Autodesk Inventor part; units mm, degrees
ref_plane "Plano de trabajo1" through (0, 0, 0) normal (0, 0, 1) x (1, 0, 0)
ref_plane "YZ Plane" through (0, 0, 0) normal (1, 0, 0) x (0, 1, 0)
ref_plane "XZ Plane" through (0, 0, 0) normal (0, 1, 0) x (-1, 0, 0)
ref_plane "Plano de trabajo1" through (0, 0, 0) normal (0, 0, 1) x (1, 0, 0)
sketch "Boceto1" plane through (0, 0, 0) normal (0, 0, 1) x (1, 0, 0)
  circle A0 centre (-10, -5) radius 1.5 construction
  line L0 (-11, -2.5) -> (-9, -2.5)
  line L1 (-7.5, -4) -> (-7.5, -6)
  line L2 (-9, -7.5) -> (-11, -7.5)
  line L3 (-12.5, -6) -> (-12.5, -4)
  line L4 (-12.5, -2.5) -> (-7.5, -7.5) construction
  line L5 (-7.5, -2.5) -> (-12.5, -7.5) construction
  arc A1 (-9, -7.5) -> (-7.5, -6) centre (-9, -6) ccw
  arc A2 (-12.5, -6) -> (-11, -7.5) centre (-11, -6) ccw
  arc A3 (-7.5, -4) -> (-9, -2.5) centre (-9, -4) ccw
  arc A4 (-11, -2.5) -> (-12.5, -4) centre (-11, -4) ccw
  circle A5 centre (-10, -5) radius 1.4
  point P0 (0, 0)
  dimension "d0" = 5
  dimension "d1" = 5
  dimension "d2" = 1.5
  dimension "d5" = 0.1
extrude "Extrusión1" add sketch "Boceto1" along normal blind 5
properties part number "ReyenedorTornillo3M"
Input: part model. Units: mm. Frame: model coordinates. Give positions to 0.01 mm unless a question says otherwise; leave off trailing zeros. Order: outer loops, then holes, each group sorted by start corner. A loop starts at its lowest first (then second) coordinate and runs counter-clockwise, first axis right, second up. Notation, with made-up numbers: M -21,70 L -14,70 A21 cw -14,76 Z; hole C 31,61.5 d3. An arc over 180 degrees is marked long. Return JSON: item names as keys, results as strings.
1) Mould query, pull axis X, two halves, no side actions, for faces 1 (the face through (-7.95, -2.93, 2.46)), 2 (the face through (-11.1, -6.1, 0)), 3 (the face through (-11.4, -5.06, 2.46)). Classes: released by +X, released by -X, zero draft, split by the parting line, or undercut.
Taken from the geometry:
{"face 1": "released by +X", "face 2": "zero draft", "face 3": "undercut"}
2) Section query D-D on x = -12. Output: boundary loops of the cut face in (y, z).
Taken from the geometry:
{"outline": "M -7.12,0 L -2.88,0 L -2.88,5 L -7.12,5 Z"}
3) Section query A-A on y = -5. Output: boundary loops of the cut face in (x, z), and give its area (3 significant figures).
Taken from the geometry:
{"outline": "M -12.5,0 L -11.4,0 L -11.4,5 L -12.5,5 Z; M -8.6,0 L -7.5,0 L -7.5,5 L -8.6,5 Z", "area": "11.0 mm2"}
4) Section query B-B on x = -10. Output: boundary loops of the cut face in (y, z), and give its area (3 significant figures).
Taken from the geometry:
{"outline": "M -7.5,0 L -6.4,0 L -6.4,5 L -7.5,5 Z; M -3.6,0 L -2.5,0 L -2.5,5 L -3.6,5 Z", "area": "11.0 mm2"}
5) Line query: L1, parallel to Y at x = -10, z = 1.8; L2, parallel to X at y = -4.95, z = 4.75; L3, parallel to X at y = -4.35, z = 3.55. Output: solid intervals per line, ascending. Write a range as [from, to].
Taken from the geometry:
{"L1": "y = [-7.5, -6.4], [-3.6, -2.5]", "L2": "x = [-12.5, -11.4], [-8.6, -7.5]", "L3": "x = [-12.5, -11.24], [-8.76, -7.5]"}
6) Section query C-C on z = 2.3. Output: boundary loops of the cut face in (x, y), and give its area (3 significant figures).
Taken from the geometry:
{"outline": "M -12.5,-6 A1.5 ccw -11,-7.5 L -9,-7.5 A1.5 ccw -7.5,-6 L -7.5,-4 A1.5 ccw -9,-2.5 L -11,-2.5 A1.5 ccw -12.5,-4 Z; hole C -10,-5 d2.8", "area": "16.9 mm2"}
